Autodesk Inventor part; units mm, degrees
ref_plane "YZ Plane" through (0, 0, 0) normal (1, 0, 0) x (0, 1, 0)
ref_plane "XZ Plane" through (0, 0, 0) normal (0, 1, 0) x (-1, 0, 0)
ref_plane "XY Plane" through (0, 0, 0) normal (0, 0, 1) x (1, 0, 0)
sketch "Boceto1" plane through (0, 0, 0) normal (0, 0, 1) x (1, 0, 0)
  circle A0 centre (0, 0) radius 55
extrude "Extrusión1" add sketch "Boceto1" against normal blind 3
sketch "Boceto2" plane through (0, 0, 0) normal (0, 0, 1) x (1, 0, 0)
  circle A0 centre (0, 0) radius 4.5
hole "Agujero1" at (0, 0, 0) direction (0, 0, -1) diameter 9 end through all
sketch "Boceto3" plane through (0, 0, 0) normal (0, 0, 1) x (1, 0, 0)
  line L0 (0, 0) -> (-11.5, 0)
  circle A0 centre (-11.5, 6.75) radius 1.25
  circle A1 centre (11.5, 6.75) radius 1.25
  circle A2 centre (11.5, -6.75) radius 1.25
  circle A3 centre (-11.5, -6.75) radius 1.25
hole "Agujero2" at (11.5, -6.75, 0) at (-11.5, 6.75, 0) at (-11.5, -6.75, 0) at (11.5, 6.75, 0) direction (0, 0, -1) diameter 2.5 end through all
sketch "Boceto4" plane through (0, 0, -3) normal (0, 0, -1) x (-1, 0, 0)
  point P0 (0, 0)
properties part number "Base2"
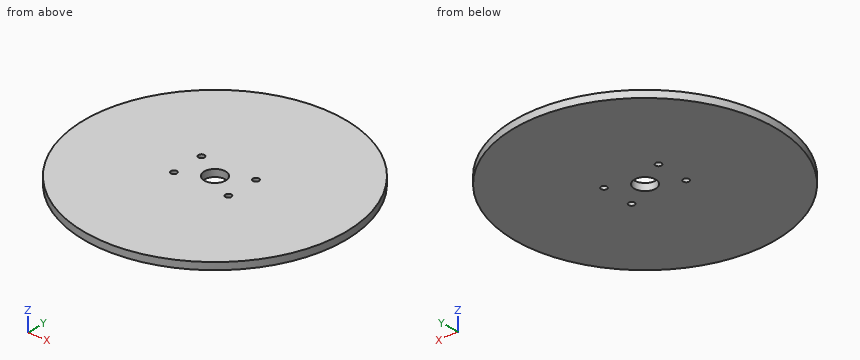
Can you work these out from the model? Positions are in its coordinate system, mm. Round coordinates to 2 decimals unless told otherwise and drop trailing zeros. Order: outer loops, then holes, each group sorted by start corner. A loop starts at its lowest first (then second) coordinate and runs counter-clockwise, first axis right, second up.
(1) If we section it at C-C (z = -1.3): Please give me the cut outline in (x, y), plus the area to 3 significant figures.
Results are:
outline: circle Ø110 at (0, 0); hole circle Ø2.5 at (-11.5, -6.75); hole circle Ø2.5 at (-11.5, 6.75); hole circle Ø9 at (0, 0); hole circle Ø2.5 at (11.5, -6.75); hole circle Ø2.5 at (11.5, 6.75)
area: 9,420 mm2
(2) If we section it at A-A (y = 0): Please give me the cut outline in (x, z), plus the area to 3 significant figures.
Results are:
outline: (-55, -3) - (-4.5, -3) - (-4.5, 0) - (-55, 0) - close; (4.5, -3) - (55, -3) - (55, 0) - (4.5, 0) - close
area: 303 mm2
(3) If I drill on L1, parallel to Y at x = 11.5, z = -1.25; L2, parallel to X at y = -6, z = -2.3; L3, parallel to X at y = -6.75, z = -1.95, over which ranges is the centre line in solid material (lowest first)?
Results are:
L1: y = -53.78 to -8, -5.5 to 5.5, 8 to 53.78
L2: x = -54.67 to -12.5, -10.5 to 10.5, 12.5 to 54.67
L3: x = -54.58 to -12.75, -10.25 to 10.25, 12.75 to 54.58
(4) If we section it at D-D (x = -11.5): Please give me the cut outline in (y, z), plus the area to 3 significant figures.
Results are:
outline: (-53.78, -3) - (-8, -3) - (-8, 0) - (-53.78, 0) - close; (-5.5, -3) - (5.5, -3) - (5.5, 0) - (-5.5, 0) - close; (8, -3) - (53.78, -3) - (53.78, 0) - (8, 0) - close
area: 308 mm2
(5) I'm going to push a flat-ended pin straight in: pin 1 (8 mm diameter, centred on x = 0, y = 0, fed in from +Z). Where does the tip first touch, or does it pass through?
Results are:
pin 1: passes through
